Source: CAD feature listing. Evaluate the final solid. Frame: model axes, mm. Face numbers are marked on the shaded views. A direction names the side the tool comes from. Round coordinates to 2 decimals unless told otherwise and drop trailing zeros. Loops run counter-clockwise (first coordinate to the right, second up) from the corner with the lowest first, then second, coordinate; pieces in that order, holes last. Notation, with made-up numbers: (48.25, -36) -> (59.25, -36) arc R29 cw to (59.25, -16) -> close; hole circle Ø1 at (4.25, 71.5). An arc over 180 degrees is marked (long way). Write item = value, one per line.
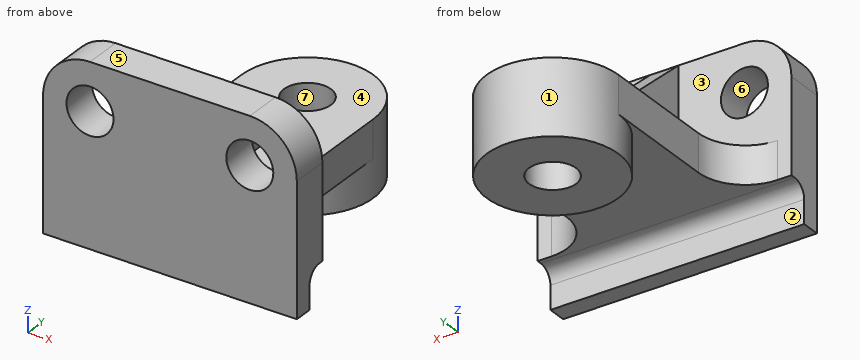
from build123d import *

# Parameters (mm, degrees)
BOSS_EXTRUDE1_DEPTH = 54
FILLET1_R           = 10
SKETCH2_R           = 5
CUT_EXTRUDE1_DEPTH  = 67.513156593
BOSS_EXTRUDE2_DEPTH = 8
FILLET2_R           = 10
BOSS_EXTRUDE3_START = 8
SKETCH4_R           = 14
BOSS_EXTRUDE3_DEPTH = 8
SKETCH5_R           = 5
CUT_EXTRUDE2_DEPTH  = 88.229582138
RIB1_REACH          = 75.634
SKETCH6_WALL_W      = 182.57011395
SKETCH6_WALL_H      = 6


with BuildPart() as part:
    # Sketch1 → Boss-Extrude1 (new body)
    with BuildSketch(Plane(origin=(0, 0, 0), x_dir=(0, 0, -1), z_dir=(1, 0, 0))):
        with BuildLine():
            Line((30, 8), (30, 7))
            ThreePointArc((30, 7), (30.878679656, 4.878679656), (33, 4))
            Line((33, 4), (38, 4))
            Line((38, 4), (38, 0))
            Line((38, 0), (0, 0))
            Line((0, 0), (0, 8))
            Line((0, 8), (30, 8))
        make_face()
    extrude(amount=-BOSS_EXTRUDE1_DEPTH)

    # Fillet1
    fillet1_edges = [part.edges().sort_by_distance(p)[0] for p in [
        (0, 4, 0),
        (-54, 4, 0),
    ]]
    fillet(fillet1_edges, radius=FILLET1_R)

    # Sketch2 → Cut-Extrude1 (cut, through all)
    with BuildSketch(Plane(origin=(0, 8, 0), x_dir=(1, 0, 0), z_dir=(0, 1, 0))):
        with Locations(Location((-44, 10, 0), (0, 0, 270))):
            Circle(SKETCH2_R)
        with Locations(Location((-10, 10, 0), (0, 0, 270))):
            Circle(SKETCH2_R)
    extrude(amount=-CUT_EXTRUDE1_DEPTH, mode=Mode.SUBTRACT)

    # Sketch3 → Boss-Extrude2 (add)
    with BuildSketch(Plane(origin=(0, 0, -30), x_dir=(-1, 0, 0), z_dir=(0, 0, -1))):
        with BuildLine():
            Line((13, 8), (41, 8))
            Line((41, 8), (41, 43))
            ThreePointArc((41, 43), (27, 57), (13, 43))
            Line((13, 43), (13, 8))
        make_face()
    extrude(amount=-BOSS_EXTRUDE2_DEPTH)

    # Fillet2
    fillet2_edges = [part.edges().sort_by_distance(p)[0] for p in [
        (-41, 8, -26),
        (-13, 8, -26),
    ]]
    fillet(fillet2_edges, radius=FILLET2_R)

    # Sketch4 → Boss-Extrude3 (add)
    with BuildSketch(Plane(origin=(0, 0, -30), x_dir=(-1, 0, 0), z_dir=(0, 0, -1)).offset(BOSS_EXTRUDE3_START)):
        with Locations((27, 43)):
            Circle(SKETCH4_R)
    extrude(amount=-BOSS_EXTRUDE3_DEPTH)

    # Sketch5 → Cut-Extrude2 (cut, through all)
    with BuildSketch(Plane(origin=(0, 0, -38), x_dir=(-1, 0, 0), z_dir=(0, 0, -1))):
        with Locations((27, 43)):
            Circle(SKETCH5_R)
    extrude(amount=-CUT_EXTRUDE2_DEPTH, mode=Mode.SUBTRACT)

    # Sketch6 wall → Rib1 (add, up to next)
    with BuildSketch(Plane(origin=(-27, 20.5, -11), x_dir=(0, 0.750713516923, -0.660627894892), z_dir=(0, 0.660627894892, 0.750713516923)), mode=Mode.PRIVATE) as rib1_sk1:
        Rectangle(SKETCH6_WALL_W, SKETCH6_WALL_H)
    rib1_tool1 = extrude(rib1_sk1.sketch, amount=-RIB1_REACH, mode=Mode.PRIVATE) - part.part
    add(rib1_tool1.solids().sort_by_distance((-27, 20.5, -11))[0])


solid = part.part
1. Section query D-D (z = -29). Return the cut outline in (x, y), then the cut area to 3 significant figures.
Evaluation:
outline = (-54, 0) -> (0, 0) -> (0, 8) -> (-3, 8) arc R10 cw to (-13, 18) -> (-13, 43) arc R14 ccw to (-41, 43) -> (-41, 18) arc R10 cw to (-51, 8) -> (-54, 8) -> close; hole circle Ø10 at (-27, 43)
area = 1,680 mm²
2. Line query: probe 1 along Y at (x, z) = (-27, -33.75); probe 2 along Y at (x, z) = (-27, -31.25); probe 3 along Z at (x, y) = (-22, 14.5). Output: solid intervals per line, ascending. Write a range as from..to.
Evaluation:
probe_1 = 0..4, 29..38, 48..57
probe_2 = 0..4.56, 29..38, 48..57
probe_3 = -30..-22
3. Set-up query: the marked faces 1, 2, 3 and 4. Return all of +Z, -Z, +X, -X, +Y, -Y with unobstructed straight access to the full face (end or side cutting, diameter ignored); none if empty.
Evaluation:
face_1 = -Z
face_2 = -Z, +X, -X
face_3 = +Z, -X, +Y
face_4 = +Z, +Y
4. Section query C-C (y = 46). Return the cut outline in (x, z), then the cut area to 3 significant figures.
Evaluation:
outline = (-40.67, -38) -> (-31, -38) -> (-31, -22) -> (-40.67, -22) -> close; (-23, -38) -> (-13.33, -38) -> (-13.33, -22) -> (-23, -22) -> close
area = 310 mm²
5. Contact query for flat-ended pins moving along their axis: pin 1 Ø11 at (y, z) = (19.5, -11.5) entering from +X; pin 2 Ø4 at (x, z) = (-47.5, -22.5) entering from -Y; pin 3 Ø4 at (y, z) = (30.5, -26) entering from +X; pin 4 Ø5 at (x, y) = (-31.5, 40.5) entering from +Z. Output: stop coordinate, or through.
Evaluation:
pin_1 = -24
pin_2 = 0
pin_3 = -13
pin_4 = -22
6. Mould query, pull axis Z, two halves, no side actions, for the marked faces 5, 6 and 7. Classes: released by +Z, released by -Z, zero draft, split by the parting line, or undercut.
Evaluation:
face_5 = released by +Z
face_6 = undercut
face_7 = zero draft
7. Section query B-B (z = -34.5). Return the cut outline in (x, y), then the cut area to 3 significant figures.
Evaluation:
outline = (-54, 0) -> (0, 0) -> (0, 4) -> (-54, 4) -> close; circle Ø28 at (-27, 43); hole circle Ø10 at (-27, 43)
area = 753 mm²
8. Section query A-A (x = -27). Return the cut outline in (y, z), then the cut area to 3 significant figures.
Evaluation:
outline = (0, -38) -> (4, -38) -> (4, -33) arc R3 cw to (7, -30) -> (29, -30) -> (29, -38) -> (38, -38) -> (38, -22) -> (33, -22) -> (8, 0) -> (0, 0) -> close; (48, -38) -> (57, -38) -> (57, -22) -> (48, -22) -> close
area = 1,000 mm²
